from build123d import *

# Parameters (mm, degrees)
SKETCH2_W                = 75
SKETCH2_H                = 75
SKETCH2_R                = 21
BOSS_EXTRUDE1_DEPTH      = 6
M4_CLEARANCE_HOLE1_D     = 4.8
M4_CLEARANCE_HOLE1_DEPTH = 25
FILLET1_R                = 6.35
SKETCH5_R                = 22.809118079
BOSS_EXTRUDE2_DEPTH      = 19
FILLET2_R                = 10
M5_TAPPED_HOLE1_D        = 4.2
M5_TAPPED_HOLE1_DEPTH    = 12.4
M5_TAPPED_HOLE1_TIP      = 1.2618073
SKETCH11_R               = 18.5
SKETCH11_R_2             = 2.1
BOSS_EXTRUDE3_DEPTH      = 27


with BuildPart() as part:
    # Sketch1 → Revolve1 (revolve)
    with BuildSketch(Plane.XY, mode=Mode.PRIVATE) as revolve1_sk:
        Polygon((-16.5, 0), (-34, 0), (-34, 6), (-24, 6), (-24, 25), (-18.5, 25), (-18.5, 13), (-16.5, 13), align=None)
    revolve(revolve1_sk.sketch.rotate(Axis((0, 0, 0), (0, 1, 0)), 270), axis=Axis((0, 0, 0), (0, 1, 0)))

    # Sketch2 → Boss-Extrude1 (add)
    with BuildSketch(Plane(origin=(0, 6, 0), x_dir=(1, 0, 0), z_dir=(0, 1, 0))):
        Rectangle(SKETCH2_W, SKETCH2_H)
        Circle(SKETCH2_R, mode=Mode.SUBTRACT)
    extrude(amount=-BOSS_EXTRUDE1_DEPTH)

    # M4 Clearance Hole1
    with Locations(Plane(origin=(0, 0, 0), x_dir=(-1, 0, 0), z_dir=(0, -1, 0))):
        with Locations((0, 0), (-31.819805153, 31.819805153), (31.819805153, 31.819805153), (31.819805153, -31.819805153), (-31.819805153, -31.819805153)):
            Hole(M4_CLEARANCE_HOLE1_D / 2, depth=M4_CLEARANCE_HOLE1_DEPTH)

    # Fillet1
    fillet1_edges = [part.edges().sort_by_distance(p)[0] for p in [
        (37.5, 3, 37.5),
        (37.5, 3, -37.5),
        (-37.5, 3, -37.5),
        (-37.5, 3, 37.5),
    ]]
    fillet(fillet1_edges, radius=FILLET1_R)

    # Sketch5 → Boss-Extrude2 (add)
    with BuildSketch(Plane(origin=(0, 25, 0), x_dir=(1, 0, 0), z_dir=(0, 1, 0))):
        with BuildLine():
            Line((0, 24), (6.5, 24))
            Line((6.5, 24), (30.5, 24))
            Line((30.5, 24), (30.5, -24))
            Line((30.5, -24), (6.5, -24))
            Line((6.5, -24), (0, -24))
            ThreePointArc((0, -24), (-24, 0), (0, 24))
        make_face()
        Circle(SKETCH5_R, mode=Mode.SUBTRACT)
    extrude(amount=-BOSS_EXTRUDE2_DEPTH)

    # Fillet2
    fillet2_edges = [part.edges().sort_by_distance(p)[0] for p in [
        (30.5, 15.5, -24),
        (30.5, 15.5, 24),
    ]]
    fillet(fillet2_edges, radius=FILLET2_R)

    # M5 Tapped Hole1
    with Locations(Plane(origin=(0, 25, 0), x_dir=(1, 0, 0), z_dir=(0, 1, 0))):
        with Locations((22.5, 16), (22.5, -16)):
            Hole(M5_TAPPED_HOLE1_D / 2, depth=M5_TAPPED_HOLE1_DEPTH)
            with Locations((0, 0, -(M5_TAPPED_HOLE1_DEPTH + M5_TAPPED_HOLE1_TIP / 2))):  # 118° drill point
                Cone(0, M5_TAPPED_HOLE1_D / 2, M5_TAPPED_HOLE1_TIP, mode=Mode.SUBTRACT)

    # Sketch11 → Boss-Extrude3 (add)
    with BuildSketch(Plane(origin=(0, 25, 0), x_dir=(1, 0, 0), z_dir=(0, 1, 0))):
        with BuildLine():
            Line((0, -24), (20.5, -24))
            ThreePointArc((20.5, -24), (27.571067812, -21.071067812), (30.5, -14))
            Line((30.5, -14), (30.5, 14))
            ThreePointArc((30.5, 14), (27.571067812, 21.071067812), (20.5, 24))
            Line((20.5, 24), (0, 24))
            ThreePointArc((0, 24), (-24, 0), (0, -24))
        make_face()
        with Locations(Location((0, 0, 0), (0, 0, 90))):
            Circle(SKETCH11_R, mode=Mode.SUBTRACT)
        with Locations(Location((22.5, -16, 0), (0, 0, 270))):
            Circle(SKETCH11_R_2, mode=Mode.SUBTRACT)
        with Locations(Location((22.5, 16, 0), (0, 0, 270))):
            Circle(SKETCH11_R_2, mode=Mode.SUBTRACT)
    extrude(amount=BOSS_EXTRUDE3_DEPTH)


solid = part.part
Geometry: final body of the model. Coordinates: model frame, mm. A direction names the side the tool comes from. Give positions to 0.01 mm unless a question says otherwise; leave off trailing zeros. Order: outer loops, then holes, each group sorted by start corner. A loop starts at its lowest first (then second) coordinate and runs counter-clockwise, first axis right, second up. Notation, with made-up numbers: (56, -30) -> (103, -30) arc R10 ccw to (103, -24) -> close; hole circle Ø6 at (61.5, -6). An arc over 180 degrees is marked (long way). Answer as a JSON object with one key per item and string values.
Q1. Draft query along Z for faces 4 (the cylindrical face through (-30.53, 3.042, 29.796)), 5 (the flat face through (0, 3, -37.5)), 6 (the flat face through (37.5, 3, 0)). Return one class per face: released by +Z, released by -Z, zero draft, split by the parting line, or undercut.
Entries:
{"face 4": "undercut", "face 5": "released by -Z", "face 6": "zero draft"}
Q2. Material intervals for probe 1 along Z at (x, y) = (21, 34); probe 2 along X at (y, z) = (40, 16); probe 3 along Y at (x, z) = (5.5, -29), sorted ascending.
Entries:
{"probe 1": "z = -23.99 to -17.47, -14.53 to 14.53, 17.47 to 23.99", "probe 2": "x = -17.89 to -9.29, 9.29 to 20.4, 24.6 to 30.3", "probe 3": "y = 0 to 6"}
Q3. Access query for faces 1 (the flat face through (0, 13, 17)), 2 (the flat face through (10, 29, 24)), 3 (the flat face through (0, 3, 37.5)). Directions: +Z, -Z, +X, -X, +Y, -Y. A direction counts if a zero-diameter tool reaches every point of the face in a straight line with its end or side. Return the directions, or none.
Entries:
{"face 1": "+Y", "face 2": "+Z, +X, -X, +Y", "face 3": "+Z, +X, -X, +Y, -Y"}
Q4. First-contact query: pin 1 (16.5 mm diameter, centred on x = 10.5, y = 25, fed in from +Z); pin 2 (1 mm diameter, centred on x = 21.5, y = 44.5, fed in from -Z); pin 3 (4 mm diameter, centred on x = 22.5, z = -16, fed in from +Y); pin 4 (4.5 mm diameter, centred on x = 31.82, z = -31.82, fed in from +Y). Flat tips, straight axial feed; report the tip coordinate or a pass-through.
Entries:
{"pin 1": "stops at z = 24", "pin 2": "stops at z = -23.99", "pin 3": "stops at y = 12.54", "pin 4": "passes through"}
Q5. Section A-A (y = 31.5). Output: boundary loops of the cut face in (x, z).
Entries:
{"outline": "(0, -24) -> (20.5, -24) arc R10 ccw to (30.5, -14) -> (30.5, 14) arc R10 ccw to (20.5, 24) -> (0, 24) arc R24 ccw to start; hole circle Ø37 at (0, 0); hole circle Ø4.2 at (22.5, -16); hole circle Ø4.2 at (22.5, 16)"}
Q6. Section C-C (z = 0). Output: boundary loops of the cut face in (x, y), plus the area to 4 significant figures.
Entries:
{"outline": "(-37.5, 0) -> (-16.5, 0) -> (-16.5, 13) -> (-18.5, 13) -> (-18.5, 52) -> (-24, 52) -> (-24, 6) -> (-37.5, 6) -> close; (16.5, 0) -> (37.5, 0) -> (37.5, 6) -> (30.5, 6) -> (30.5, 52) -> (18.5, 52) -> (18.5, 13) -> (16.5, 13) -> close", "area": "1,085 mm^2"}
Q7. Section B-B (x = 14.5). Output: boundary loops of the cut face in (y, z), plus the area to 3 significant figures.
Entries:
{"outline": "(0, -37.5) -> (6, -37.5) -> (6, -24) -> (52, -24) -> (52, -11.49) -> (13, -11.49) -> (13, -7.87) -> (0, -7.87) -> close; (0, 7.87) -> (13, 7.87) -> (13, 11.49) -> (52, 11.49) -> (52, 24) -> (6, 24) -> (6, 37.5) -> (0, 37.5) -> close", "area": "1,560 mm^2"}
Q8. Section D-D (z = -20). Output: boundary loops of the cut face in (x, y).
Entries:
{"outline": "(-37.5, 0) -> (37.5, 0) -> (37.5, 6) -> (28.5, 6) -> (28.5, 52) -> (-13.27, 52) -> (-13.27, 6) -> (-37.5, 6) -> close"}
